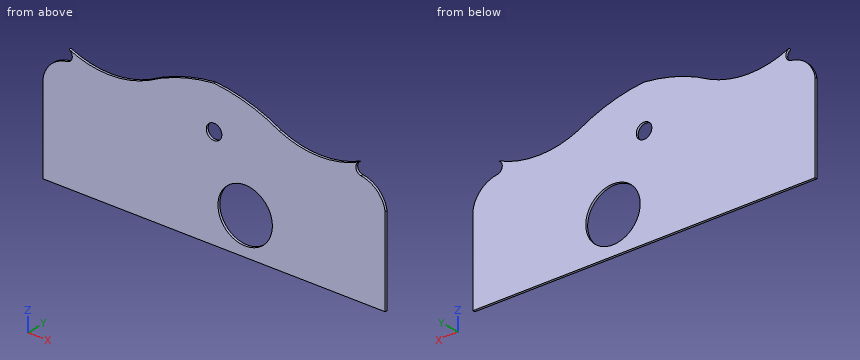
from build123d import *

# Parameters (mm, degrees)
SKETCH2_R           = 17.5
SKETCH2_R_2         = 5
BOSS_EXTRUDE2_DEPTH = 1.5


with BuildPart() as part:
    # Sketch2 → Boss-Extrude2 (new body)
    with BuildSketch(Plane(origin=(0, 22.5, 0), x_dir=(1, 0, 0), z_dir=(0, 1, 0))):
        with BuildLine():
            Line((-110, 50), (110, 50))
            Line((110, 50), (110, -7.5))
            ThreePointArc((110, -7.5), (104.755451902, -17.601037804), (94.5, -22.536820999))
            ThreePointArc((94.5, -22.536820999), (91.210601206, -25.822153148), (93.25, -30))
            ThreePointArc((93.25, -30), (67.606257623, -24.318329423), (41.962515246, -30))
            ThreePointArc((41.962515246, -30), (21.653208784, -38.627914511), (0, -42.876136156))
            ThreePointArc((0, -42.876136156), (-21.653208784, -38.627914511), (-41.962515246, -30))
            ThreePointArc((-41.962515246, -30), (-67.606257623, -24.318329423), (-93.25, -30))
            ThreePointArc((-93.25, -30), (-91.210601206, -25.822153148), (-94.5, -22.536820999))
            ThreePointArc((-94.5, -22.536820999), (-104.755451902, -17.601037804), (-110, -7.5))
            Line((-110, -7.5), (-110, 50))
        make_face()
        with Locations(Location((20, 26, 0), (0, 0, 270))):
            Circle(SKETCH2_R, mode=Mode.SUBTRACT)
        with Locations(Location((0, -15, 0), (0, 0, 270))):
            Circle(SKETCH2_R_2, mode=Mode.SUBTRACT)
    extrude(amount=BOSS_EXTRUDE2_DEPTH)


solid = part.part
Here's how the part is built. I have some questions about the finished solid (model axes, mm). Round coordinates to 2 decimals unless told otherwise and drop trailing zeros. Loops run counter-clockwise (first coordinate to the right, second up) from the corner with the lowest first, then second, coordinate; pieces in that order, holes last. Notation, with made-up numbers: (6, 76.25) -> (53, 76.25) arc R3 ccw to (53, 81.25) -> close; hole circle Ø3 at (60.25, 74.5). An arc over 180 degrees is marked (long way). Write each question's results on one line, items separated by ' | '.
(1) If we section it at A-A, the plane z = -26: List the corners of the cut face in (x, y) for me.
Worked answers:
outline: (-110, 22.5) -> (2.5, 22.5) -> (2.5, 24) -> (-110, 24) -> close; (37.5, 22.5) -> (110, 22.5) -> (110, 24) -> (37.5, 24) -> close
(2) If we section it at D-D, the plane x = -51.5: List the corners of the cut face in (y, z) for me, then the cut area to 3 significant figures.
Worked answers:
outline: (22.5, -50) -> (24, -50) -> (24, 26.49) -> (22.5, 26.49) -> close | area: 115 mm2
(3) If we section it at C-C, the plane x = 34: List the corners of the cut face in (y, z) for me, then the cut area to 3 significant figures.
Worked answers:
outline: (22.5, -50) -> (24, -50) -> (24, -36.5) -> (22.5, -36.5) -> close; (22.5, -15.5) -> (24, -15.5) -> (24, 33.98) -> (22.5, 33.98) -> close | area: 94.5 mm2
(4) If we section it at B-B, the plane y = 23.4: List the corners of the cut face in (x, z) for me.
Worked answers:
outline: (-110, -50) -> (110, -50) -> (110, 7.5) arc R18 ccw to (94.5, 22.54) arc R4 cw to (93.25, 30) arc R60.71 cw to (41.96, 30) arc R106.28 ccw to (0, 42.88) arc R106.28 ccw to (-41.96, 30) arc R60.71 cw to (-93.25, 30) arc R4 cw to (-94.5, 22.54) arc R18 ccw to (-110, 7.5) -> close; hole circle Ø10 at (0, 15); hole circle Ø35 at (20, -26)
(5) If I drill on L1, parallel to X at y = 22.7, z = -26.5; L2, parallel to X at y = 23.95, z = -32.5; L3, parallel to Z at x = 23.5, y = 23.15, over which ranges is the centre line in solid material (lowest first)?
Worked answers:
L1: -110 to 2.51, 37.49 to 110 | L2: -110 to 3.75, 36.25 to 110 | L3: -50 to -43.15, -8.85 to 38.04
